Verification items for this drawing (mm, ordinates from the low corner). A direction names the side the tool comes from. Coordinates: 2 decimals unless noted, no trailing zeros. Order: outer loops, then holes, each group sorted by start corner. A loop starts at its lowest first (then second) coordinate and runs counter-clockwise, first axis right, second up. Notation, with made-up numbers: (87, 52.5) -> (92, 52.5) arc R23 cw to (92, 72.5) -> close; hole circle Ø8 at (57, 62.25). An arc over 180 degrees is marked (long way). Put each result on its own line as item: value. Start each with the question number.
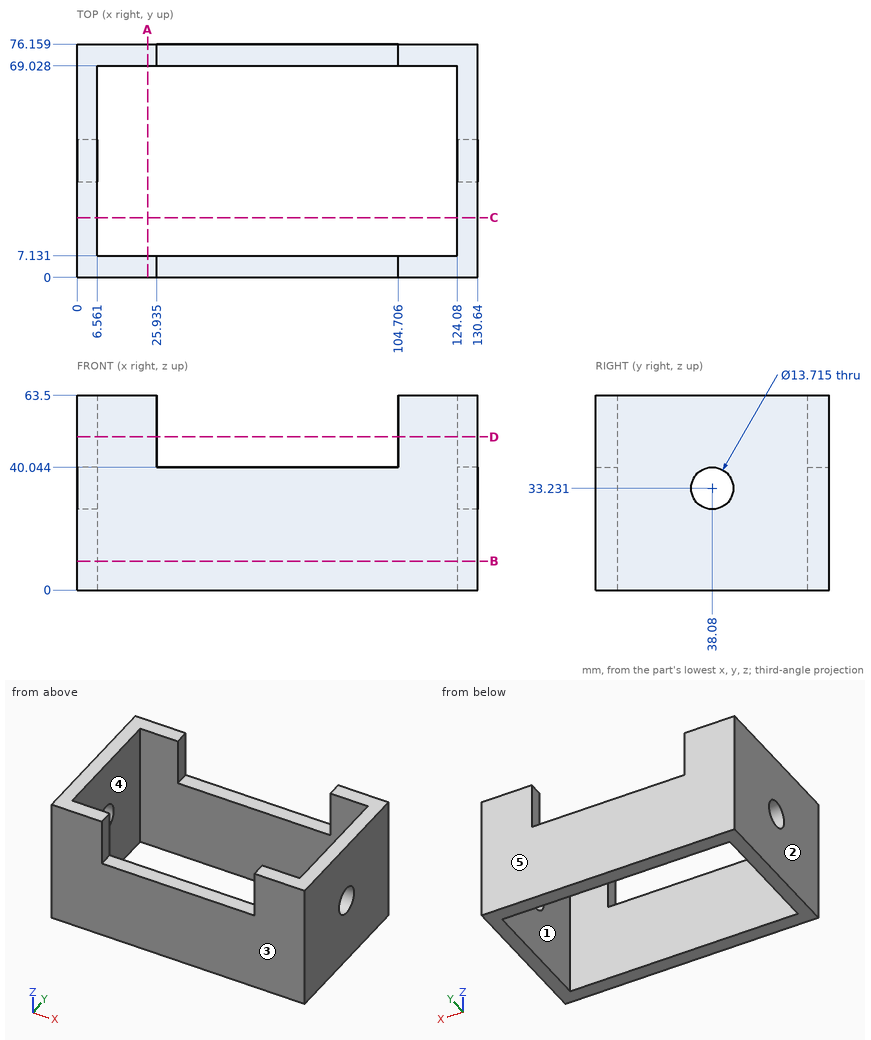
1) Sectioned sample at D-D (z = 50). Record the boundary of the cut face in (x, y) (1 decimal), plus the area to 3 significant figures.
2) Gauge pin test, flat end, axial feed: pin 1 (2 mm diameter, centred on x = 71.5, y = 5, fed in from +Z). Record the tip position at first contact, or that the pin passes through.
3) Sectioned sample at A-A (x = 23). Record the boundary of the cut face in (y, z).
4) Sectioned sample at B-B (z = 9.5). Record the boundary of the cut face in (x, y).
5) Mould release check, pull along Y, two halves, no side actions. Record for the marked faces 1, 2 and 3: +Y half, -Y half, draft (parallel to the pull), parting line (faces both ways), or undercut.
6) Access from +Z, -Z, +X, -X, +Y, -Y to the whole of each face (thin tool, end or side, straight path). Record for the marked faces 4 and 5.
7) Sectioned sample at C-C (y = 19.5). Record the boundary of the cut face in (x, z), plus the area to 3 significant figures.
8) Scan lines: line 1 along X through (y, z) = (28.5, 42); line 2 along Y through (x, z) = (64, 36.5); line 3 along Z through (x, y) = (81.5, 5) (1 decimal). Record each from-to range of solid material in increasing order. Write a range as [from, to].
Entries:
1. outline: (0, 0) -> (25.9, 0) -> (25.9, 7.1) -> (6.6, 7.1) -> (6.6, 69) -> (25.9, 69) -> (25.9, 76.2) -> (0, 76.2) -> close; (104.7, 0) -> (130.6, 0) -> (130.6, 76.2) -> (104.7, 76.2) -> (104.7, 69) -> (124.1, 69) -> (124.1, 7.1) -> (104.7, 7.1) -> close
1. area: 1,550 mm2
2. pin 1: stops at z = 40.04
3. outline: (0, 0) -> (7.13, 0) -> (7.13, 63.5) -> (0, 63.5) -> close; (69.03, 0) -> (76.16, 0) -> (76.16, 63.5) -> (69.03, 63.5) -> close
4. outline: (0, 0) -> (130.64, 0) -> (130.64, 76.16) -> (0, 76.16) -> close; hole (6.56, 7.13) -> (124.08, 7.13) -> (124.08, 69.03) -> (6.56, 69.03) -> close
5. face 1: undercut
5. face 2: draft
5. face 3: -Y half
6. face 4: +Z, -Z
6. face 5: +Z, -Z, +X, -X, +Y
7. outline: (0, 0) -> (6.56, 0) -> (6.56, 63.5) -> (0, 63.5) -> close; (124.08, 0) -> (130.64, 0) -> (130.64, 63.5) -> (124.08, 63.5) -> close
7. area: 833 mm2
8. line 1: x = [0, 6.56], [124.08, 130.64]
8. line 2: y = [0, 7.13], [69.03, 76.16]
8. line 3: z = [0, 40]
